Geometry: see drawing. Coordinates: mm, zero at the bounding-box minimum. A direction names the side the tool comes from. Coordinates: 2 decimals unless noted, no trailing zeros. Write each loop counter-clockwise with the first axis right and the second up, starting at its lowest first coordinate (ties: lowest second). Pieces come first, ordered by that corner, then holes.
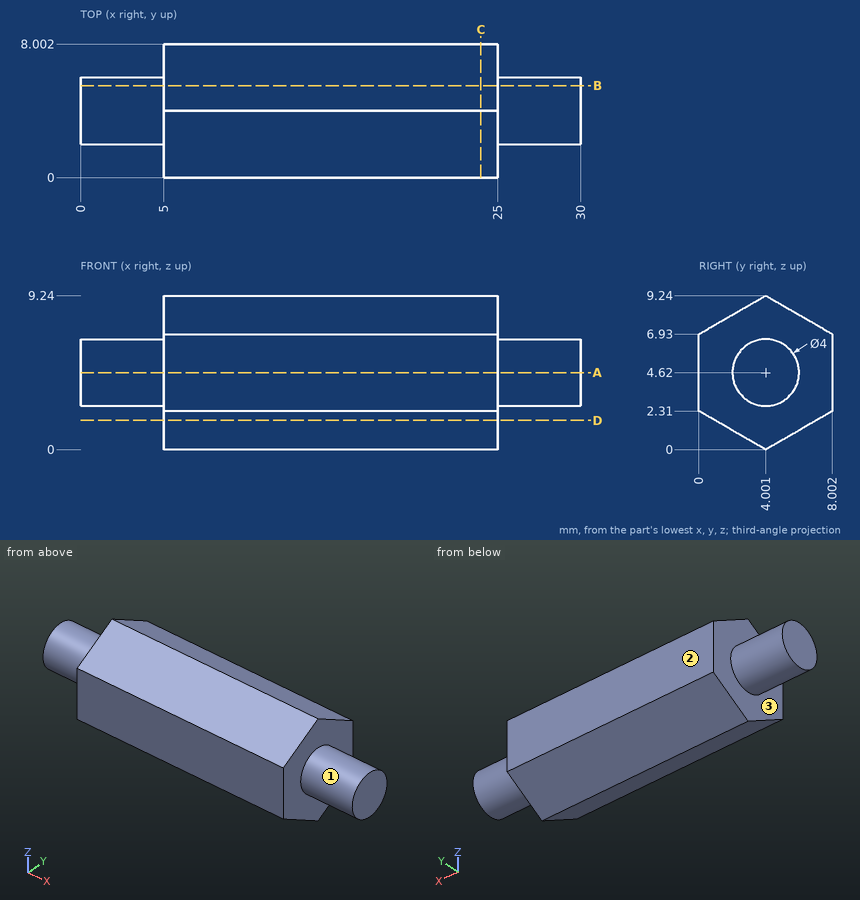
Item 1: Section B-B, the plane y = 5.5. Output: boundary loops of the cut face in (x, z).
Derived:
outline: (0, 3.3) - (5, 3.3) - (5, 0.87) - (25, 0.87) - (25, 3.3) - (30, 3.3) - (30, 5.94) - (25, 5.94) - (25, 8.37) - (5, 8.37) - (5, 5.94) - (0, 5.94) - close
Item 2: Section C-C, the plane x = 24. Output: boundary loops of the cut face in (y, z), plus the area to 3 significant figures.
Derived:
outline: (0, 2.31) - (4, 0) - (8, 2.31) - (8, 6.93) - (4, 9.24) - (0, 6.93) - close
area: 55.5 mm2
Item 3: Set-up query: the marked faces 1, 2 and 3. Return all of +Z, -Z, +X, -X, +Y, -Y with unobstructed straight access to the full face (end or side cutting, diameter ignored); none if empty.
Derived:
face 1: +X
face 2: +Z, -Z, +X, -X, +Y
face 3: -X
Item 4: Section A-A, the plane z = 4.62. Output: boundary loops of the cut face in (x, y), plus the area to 3 significant figures.
Derived:
outline: (0, 2) - (5, 2) - (5, 0) - (25, 0) - (25, 2) - (30, 2) - (30, 6) - (25, 6) - (25, 8) - (5, 8) - (5, 6) - (0, 6) - close
area: 200 mm2
Item 5: Material intervals for probe 1 along X at (y, z) = (0.5, 2.25); probe 2 along Z at (x, y) = (28, 4.5); probe 3 along Z at (x, y) = (11.75, 2.75), sorted ascending.
Derived:
probe 1: x = 5 to 25
probe 2: z = 2.68 to 6.56
probe 3: z = 0.72 to 8.52
Item 6: Section D-D, the plane z = 1.75. Output: boundary loops of the cut face in (x, y), plus the area to 3 significant figures.
Derived:
outline: (5, 0.97) - (25, 0.97) - (25, 7.03) - (5, 7.03) - close
area: 121 mm2
Item 7: Pin query (flat end, axial travel): pin 1 (4 mm diameter, centred on x = 9, z = 4, fed in from -Y); pin 2 (3 mm diameter, centred on x = 22, y = 3, fed in from +Z); pin 3 (4 mm diameter, centred on x = 3.5, y = 2, fed in from -Z); pin 4 (2 mm diameter, centred on y = 5, z = 1.5, fed in from +X). Return the tip coordinate at first contact, or that it passes through.
Derived:
pin 1: stops at y = 0
pin 2: stops at z = 9.24
pin 3: stops at z = 0.39
pin 4: stops at x = 25
